Geometry check sheet. Reference: drawing and pictorial views, mm from the part's lowest x, y, z. Give positions to 0.01 mm unless a question says otherwise; leave off trailing zeros. Order: outer loops, then holes, each group sorted by start corner. A loop starts at its lowest first (then second) coordinate and runs counter-clockwise, first axis right, second up. Notation, with made-up numbers: (-20, 22.5) - (-8, 22.5) arc R15 ccw to (-8, 40.5) - close; hole circle Ø7 at (63, 52). An arc over 180 degrees is marked (long way). Answer in a Markdown table with one row per item.
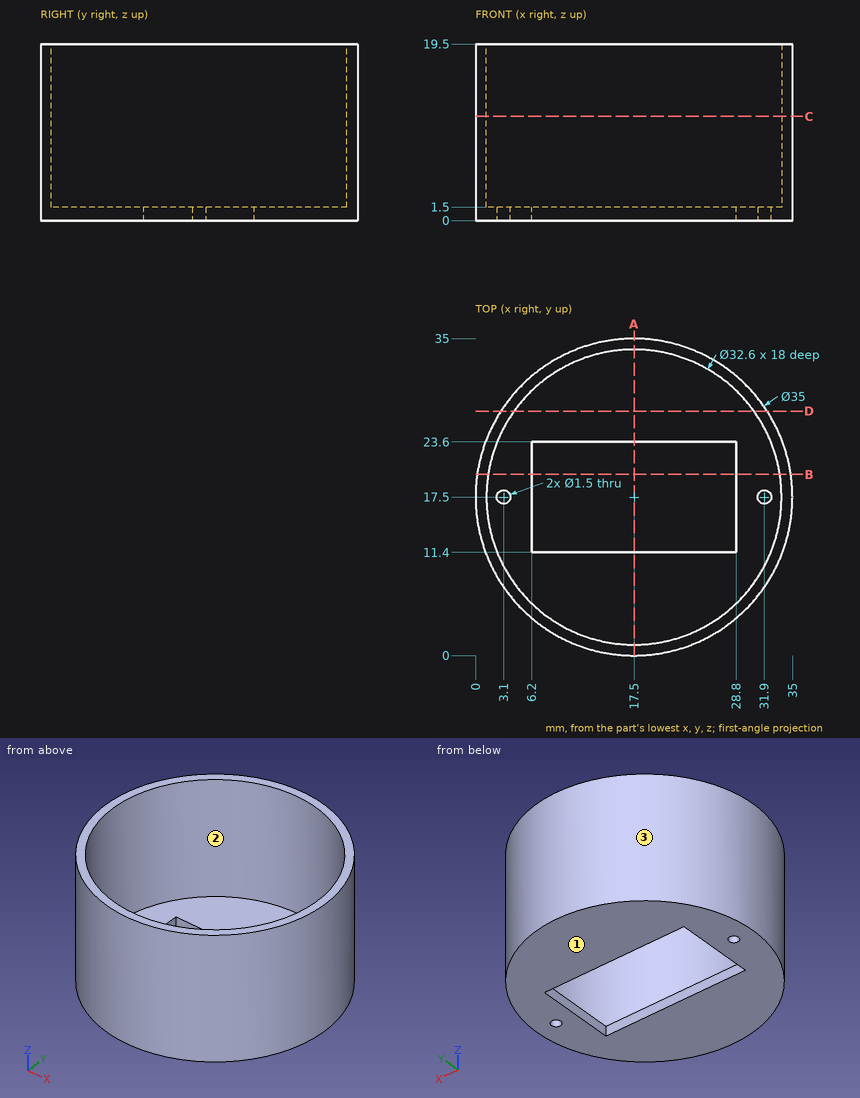
(1) Thickness scan on L1, parallel to Y at x = 17.5, z = 13.75; L2, parallel to Z at x = 13, y = 28; L3, parallel to Y at x = 5, z = 7. Record the ranges inside material, lowest first.
Geometry says:
| item | result |
|---|---|
| L1 | 0 to 1.2, 33.8 to 35 |
| L2 | 0 to 1.5 |
| L3 | 5.25 to 7.04, 27.96 to 29.75 |
(2) Cross-section at D-D, the plane y = 27. Record the cut outline in (x, z).
Geometry says:
| item | result |
|---|---|
| outline | (2.8, 0) - (32.2, 0) - (32.2, 19.5) - (30.75, 19.5) - (30.75, 1.5) - (4.25, 1.5) - (4.25, 19.5) - (2.8, 19.5) - close |
(3) Mould release check, pull along Y, two halves, no side actions. Record for the marked faces 1, 2 and 3: pulls with the +Y half, pulls with the -Y half, needs draft (parallel to the pull), parting line crosses it, or undercut.
Geometry says:
| item | result |
|---|---|
| face 1 | needs draft |
| face 2 | undercut |
| face 3 | parting line crosses it |
(4) Cross-section at A-A, the plane x = 17.5. Record the cut outline in (y, z).
Geometry says:
| item | result |
|---|---|
| outline | (0, 0) - (11.4, 0) - (11.4, 1.5) - (1.2, 1.5) - (1.2, 19.5) - (0, 19.5) - close; (23.6, 0) - (35, 0) - (35, 19.5) - (33.8, 19.5) - (33.8, 1.5) - (23.6, 1.5) - close |
(5) Gauge pin test, flat ends, axial feed: P1, Ø1.6, axis at y = 15, z = 1, coming from the -X side; P2, Ø2.5, axis at x = 3.1, y = 17.5, coming from the -Z side; P3, Ø6, axis at x = 23.5, z = 13.5, coming from the +Y side; P4, Ø0.9, axis at x = 31.9, y = 17.5, coming from the +Z side. Record the tip position at first contact, or that the pin passes through.
Geometry says:
| item | result |
|---|---|
| P1 | x = 0.08 |
| P2 | z = 0 |
| P3 | y = 34.74 |
| P4 | through |
(6) Cross-section at C-C, the plane z = 11.5. Record the cut outline in (x, y), then the cut area to 3 significant figures.
Geometry says:
| item | result |
|---|---|
| outline | circle Ø35 at (17.5, 17.5); hole circle Ø32.6 at (17.5, 17.5) |
| area | 127 mm² |
(7) Cross-section at B-B, the plane y = 20. Record the cut outline in (x, z).
Geometry says:
| item | result |
|---|---|
| outline | (0.18, 0) - (6.2, 0) - (6.2, 1.5) - (1.39, 1.5) - (1.39, 19.5) - (0.18, 19.5) - close; (28.8, 0) - (34.82, 0) - (34.82, 19.5) - (33.61, 19.5) - (33.61, 1.5) - (28.8, 1.5) - close |
